```python
from build123d import *

# Parameters (mm, degrees)
CUT_EXTRUDE_1_DEPTH      = 12.5
CUT_EXTRUDE_1_DEPTH_BACK = 12.5
CUT_EXTRUDE_2_DEPTH      = 12.5
CUT_EXTRUDE_2_DEPTH_BACK = 12.5


with BuildPart() as part:
    # Sketch 1 → Revolve 1 (revolve)
    with BuildSketch(Plane(origin=(0, 0, 0), x_dir=(0, 0, -1), z_dir=(1, 0, 0))):
        Polygon((-52, 0), (-52, 10.08), (-51.08, 11), (-12, 11), (-10.5, 12.5), (854.5, 12.5), (854.5, 39.5), (899.5, 39.5), (899.5, 0), align=None)
    revolve(axis=Axis((0, 0, -899.5), (0, 0, 1)))

    # Sketch 2 → Cut-Extrude 1 (cut, two sides)
    with BuildSketch(Plane(origin=(0, 0, 0), x_dir=(1, 0, 0), z_dir=(0, 1, 0))) as cut_extrude_1_sk:
        Polygon((11, -3.9), (11, -12), (12.5, -12), (12.5, -2.4), align=None)
    extrude(amount=CUT_EXTRUDE_1_DEPTH, mode=Mode.SUBTRACT)
    extrude(cut_extrude_1_sk.sketch, amount=-CUT_EXTRUDE_1_DEPTH_BACK, mode=Mode.SUBTRACT)

    # Sketch 3 → Cut-Extrude 2 (cut, two sides)
    with BuildSketch(Plane(origin=(0, 0, 0), x_dir=(1, 0, 0), z_dir=(0, 1, 0))) as cut_extrude_2_sk:
        Polygon((-12.5, -2.4), (-12.5, -12), (-11, -12), (-11, -3.9), align=None)
    extrude(amount=CUT_EXTRUDE_2_DEPTH, mode=Mode.SUBTRACT)
    extrude(cut_extrude_2_sk.sketch, amount=-CUT_EXTRUDE_2_DEPTH_BACK, mode=Mode.SUBTRACT)


solid = part.part
```
Geometry: final body of the model. Coordinates: model frame, mm. A direction names the side the tool comes from. Coordinates: 2 decimals unless noted, no trailing zeros. Loops run counter-clockwise (first coordinate to the right, second up) from the corner with the lowest first, then second, coordinate; pieces in that order, holes last. Notation, with made-up numbers: (36.25, -27.75) -> (73.25, -27.75) arc R21 ccw to (73.25, -23.75) -> close; hole circle Ø10 at (-21.5, 65). An arc over 180 degrees is marked (long way). Use a Markdown table: item, result. Add a question column.
(1) Line query: line 1 along Z through (x, y) = (27, -5); line 2 along X through (y, z) = (-11, -442); line 3 along Y through (x, z) = (2, -356.5). Output: solid intervals per line, ascending.
(2) Access query for faces 1 (the cylindrical face through (10.74, -2.38, 31.27)), 2 (the cylindrical face through (-26.7, -29.11, -877.32)). Directions: +Z, -Z, +X, -X, +Y, -Y. A direction counts if a zero-diameter tool reaches every point of the face in a straight line with its end or side. Return the directions, or none.
(3) Pin query (flat end, axial travel): pin 1 Ø9 at (y, z) = (0.5, 9.5) entering from +X; pin 2 Ø9 at (y, z) = (-0.5, 7.5) entering from -X; pin 3 Ø2 at (x, y) = (-20, 31) entering from +Z. Return the tip coordinate at first contact, or that it passes through.
(4) Section query C-C, the plane y = -24.5. Return loops of the section in (x, z), plus the area to 3 significant figures.
(5) Section query B-B, the plane z = -214. Return loops of the section in (x, y), plus the area to 3 significant figures.
(6) Section query A-A, the plane x = 0. Return loops of the section in (y, z).
Answer:
| question | item | result |
|---|---|---|
| 1 | line 1 | z = -899.5 to -854.5 |
| 1 | line 2 | x = -5.94 to 5.94 |
| 1 | line 3 | y = -12.34 to 12.34 |
| 2 | face 1 | +Z |
| 2 | face 2 | +Z, -Z |
| 3 | pin 1 | stops at x = 11 |
| 3 | pin 2 | stops at x = -11.9 |
| 3 | pin 3 | stops at z = -854.5 |
| 4 | outline | (-30.98, -899.5) -> (30.98, -899.5) -> (30.98, -854.5) -> (-30.98, -854.5) -> close |
| 4 | area | 2,790 mm^2 |
| 5 | outline | circle Ø25 at (0, 0) |
| 5 | area | 491 mm^2 |
| 6 | outline | (-39.5, -899.5) -> (39.5, -899.5) -> (39.5, -854.5) -> (12.5, -854.5) -> (12.5, 10.5) -> (11, 12) -> (11, 51.08) -> (10.08, 52) -> (-10.08, 52) -> (-11, 51.08) -> (-11, 12) -> (-12.5, 10.5) -> (-12.5, -854.5) -> (-39.5, -854.5) -> close |
